Check sheet for the modelled part. Datum: model origin and axes. Units: mm. A direction names the side the tool comes from. Give positions to 0.01 mm unless a question says otherwise; leave off trailing zeros. Loops run counter-clockwise (first coordinate to the right, second up) from the corner with the lowest first, then second, coordinate; pieces in that order, holes last. Notation, with made-up numbers: M -16.75,70 L -0.75,70 A26 ccw -0.75,101 Z; hole C -6,51 d2. An arc over 180 degrees is marked long. Put each result on its own line as item: value. Start each with the question number.
```python
from build123d import *

# Parameters (mm, degrees)
F0_R     = 2.1
F1_DEPTH = 4
F2_SIZE  = 2
F3_R     = 3.75
F4_DEPTH = 2.5
F5_W     = 83.5
F5_H     = 19.5
F6_DEPTH = 30
F7_R     = 3


with BuildPart() as f1:
    # F0 (on Front) → F1 (new body)
    with BuildSketch(Plane.XZ):
        with BuildLine():
            Line((0, 12.7), (-46.481854, 12.7))
            ThreePointArc((-46.481854, 12.7), (-53.5, 0), (-46.481854, -12.7))
            Line((-46.481854, -12.7), (0, -12.7))
            Line((0, -12.7), (46.481854, -12.7))
            ThreePointArc((46.481854, -12.7), (53.5, 0), (46.481854, 12.7))
            Line((46.481854, 12.7), (0, 12.7))
        make_face()
        with Locations((-47, 0)):
            Circle(F0_R, mode=Mode.SUBTRACT)
        with Locations((47, 0)):
            Circle(F0_R, mode=Mode.SUBTRACT)
    extrude(amount=F1_DEPTH)

    # F2
    f2_edges = [f1.edges().sort_by_distance(p)[0] for p in [
        (0, -4, 12.7),
        (53.5, -4, 0),
        (0, -4, -12.7),
        (-53.5, -4, 0),
    ]]
    chamfer(f2_edges, length=F2_SIZE)

    # F3 (on face) → F4 (cut)
    with BuildSketch(Plane.XZ.offset(4)):
        with Locations((-47, 0)):
            Circle(F3_R)
        with Locations((47, 0)):
            Circle(F3_R)
    extrude(amount=-F4_DEPTH, mode=Mode.SUBTRACT)

    # F5 (on face) → F6 (join)
    with BuildSketch(Plane(origin=(0, 0, 0), x_dir=(-1, 0, 0), z_dir=(0, 1, 0))):
        Rectangle(F5_W, F5_H)
    extrude(amount=F6_DEPTH)

    # F7
    f7_edges = [f1.edges().sort_by_distance(p)[0] for p in [
        (41.75, 15, 9.75),
        (-41.75, 15, 9.75),
        (-41.75, 15, -9.75),
        (41.75, 15, -9.75),
    ]]
    fillet(f7_edges, radius=F7_R)


solid = f1.part
```
Q1. Access from +Z, -Z, +X, -X, +Y, -Y to the whole of each face (thin tool, end or side, straight path). Record for faces 1 (the face through (-40.89, 15.21, -8.85)), 2 (the face through (-41.75, 15, 0)), 3 (the face through (49, -1.5, -2)), 4 (the face through (0, 0, 11)), 5 (the face through (40.89, 15.21, 8.85)).
Q2. Depth check by flat-ended pin: P1, Ø5, axis at x = -47, z = 0, coming from the +Y side; P2, Ø3, axis at x = 7.5, y = 6, coming from the +Z side; P3, Ø10, axis at y = 1, z = 10, coming from the +X side. Enter the tip coordinate at first touch or a pass-through.
Q3. Section check C-C, the plane x = -32.5. Record the cut outline in (y, z).
Q4. Thickness scan on line 1 along X through (y, z) = (27.5, 4.75); line 2 along Z through (x, y) = (26.5, 6); line 3 along Y through (x, z) = (-44.5, -7.5). Record the ranges inside material, lowest first. Write a range as [from, to].
Q5. Mould release check, pull along X, two halves, no side actions. Record for faces 6 (the face through (41.75, 15, 0)), 7 (the face through (1, 15, 9.75)), 8 (the face through (43.254, -2.768, 0.165)): pulls with the +X half, pulls with the -X half, needs draft (parallel to the pull), parting line crosses it, or undercut.
Q6. Section check B-B, the plane y = 20.5. Record the cut outline in (x, z).
Q7. Section check A-A, the plane z = 0. Record the cut outline in (x, y), then the cut area to 3 significant figures.
Found:
1. face 1: -Z, -X, +Y
1. face 2: +Z, -Z, -X, +Y
1. face 3: -Y
1. face 4: +Y
1. face 5: +Z, +X, +Y
2. P1: stops at y = 0
2. P2: stops at z = 9.75
2. P3: stops at x = 52.61
3. outline: M -4,-10.7 L -2,-12.7 L 0,-12.7 L 0,-9.75 L 30,-9.75 L 30,9.75 L 0,9.75 L 0,12.7 L -2,12.7 L -4,10.7 Z
4. line 1: x = [-41.75, 41.75]
4. line 2: z = [-9.75, 9.75]
4. line 3: y = [-4, 0]
5. face 6: pulls with the +X half
5. face 7: needs draft
5. face 8: undercut
6. outline: M -41.75,-6.75 A3 ccw -38.75,-9.75 L 38.75,-9.75 A3 ccw 41.75,-6.75 L 41.75,6.75 A3 ccw 38.75,9.75 L -38.75,9.75 A3 ccw -41.75,6.75 Z
7. outline: M -53.5,-2 L -51.5,-4 L -50.75,-4 L -50.75,-1.5 L -49.1,-1.5 L -49.1,0 L -53.5,0 Z; M -44.9,-1.5 L -43.25,-1.5 L -43.25,-4 L 43.25,-4 L 43.25,-1.5 L 44.9,-1.5 L 44.9,0 L 41.75,0 L 41.75,30 L -41.75,30 L -41.75,0 L -44.9,0 Z; M 49.1,-1.5 L 50.75,-1.5 L 50.75,-4 L 51.5,-4 L 53.5,-2 L 53.5,0 L 49.1,0 Z
7. area: 2,880 mm^2
